from build123d import *

# Parameters (mm, degrees)
SKETCH_1_R          = 21
SKETCH_1_R_2        = 8
EXTRUDE_1_DEPTH     = 2
EXTRUDE_3_DEPTH     = 4
FILLET_1_R          = 1
SKETCH_3_R          = 1
CUT_EXTRUDE_2_DEPTH = 3


with BuildPart() as part:
    # Эскиз1 → Бобышка-Вытянуть1 (new body)
    with BuildSketch(Plane.XY):
        Circle(SKETCH_1_R)
        Circle(SKETCH_1_R_2, mode=Mode.SUBTRACT)
    extrude(amount=EXTRUDE_1_DEPTH)

    # Эскиз1<5> → Бобышка-Вытянуть3 (add)
    with BuildSketch(Plane.XY):
        with BuildLine():
            ThreePointArc((0, -19), (-19, 0), (0, 19))
            Line((0, 19), (0, 21))
            ThreePointArc((0, 21), (-21, 0), (0, -21))
            Line((0, -21), (0, -19))
        make_face()
        with BuildLine():
            Line((0, 21), (0, 19))
            ThreePointArc((0, 19), (13.435028843, 13.435028843), (19, 0))
            ThreePointArc((19, 0), (13.435028843, -13.435028843), (0, -19))
            Line((0, -19), (0, -21))
            ThreePointArc((0, -21), (14.849242405, -14.849242405), (21, 0))
            ThreePointArc((21, 0), (14.849242405, 14.849242405), (0, 21))
        make_face()
    extrude(amount=EXTRUDE_3_DEPTH)

    # Скругление1
    fillet_1_edges = [part.edges().sort_by_distance(p)[0] for p in [
        (0, 21, 4),
        (-21, 0, 0),
    ]]
    fillet(fillet_1_edges, radius=FILLET_1_R)

    # Эскиз3 → Вырез-Вытянуть2 (cut, through all)
    with BuildSketch(Plane.XY.offset(2)):
        with Locations((11.257055761, 6.499264174)):
            Circle(SKETCH_3_R)
        with Locations((11.257055761, -6.499264174)):
            Circle(SKETCH_3_R)
        with Locations((0, -12.998528347)):
            Circle(SKETCH_3_R)
        with Locations((-11.257055761, -6.499264174)):
            Circle(SKETCH_3_R)
        with Locations((0, 12.998528347)):
            Circle(SKETCH_3_R)
        with Locations((-11.257055761, 6.499264174)):
            Circle(SKETCH_3_R)
    extrude(amount=-CUT_EXTRUDE_2_DEPTH, mode=Mode.SUBTRACT)


solid = part.part
Verification items for the finished model (mm, model axes). A direction names the side the tool comes from. Give positions to 0.01 mm unless a question says otherwise; leave off trailing zeros. Write item = value, one per line. Start each with the question number.
Q1. Depth check by flat-ended pin: P1, Ø2.5, axis at x = -11.26, y = -6.5, coming from the +Z side; P2, Ø2, axis at x = -6.5, z = 1.5, coming from the +Y side; P3, Ø1, axis at y = -3, z = 2.5, coming from the +X side. Enter the tip coordinate at first touch or a pass-through.
Q2. Mould release check, pull along X, two halves, no side actions. Record for faces 3 (the face through (9, 0, 0)), 4 (the face through (18.516, -9.907, 2.208)), 5 (the face through (-1.73, -7.81, 0.99)): released by +X, released by -X, zero draft, split by the parting line, or undercut.
Q3. Thickness scan on line 1 (Y direction, x = 0, z = 1.05); line 2 (Y direction, x = -12, z = 1.15); line 3 (Z direction, x = -7, y = 15). Record the ranges inside material, lowest first.
Q4. Tool access check on faces 1 (the face through (8.2, 0.3, 2)), 2 (the face through (-10.333, -6.882, 1.014)). Record the directions out of +Z, -Z, +X, -X, +Y, -Y that give a thin tool (end or side, any length) a straight path to the whole face; none if there is none.
Answer key:
q1.P1 = 2
q1.P2 = 20.27
q1.P3 = 20.85
q2.face_3 = zero draft
q2.face_4 = split by the parting line
q2.face_5 = undercut
q3.line_1 = -21 to -14, -12 to -8, 8 to 12, 14 to 21
q3.line_2 = -17.23 to -7.17, -5.83 to 5.83, 7.17 to 17.23
q3.line_3 = 0 to 2
q4.face_1 = +Z
q4.face_2 = +Z, -Z
